from build123d import *

# Parameters (mm, degrees)
SKETCH1_W           = 25.4
SKETCH1_H           = 25.4
SKETCH1_W_2         = 19.05
SKETCH1_H_2         = 19.05
EXTRUDE_THIN1_DEPTH = 292.1
SKETCH4_R           = 2.4892
CUT_EXTRUDE1_DEPTH  = 26.4
CUT_EXTRUDE2_DEPTH  = 26.4
SKETCH3_R           = 3.175
CUT_EXTRUDE3_DEPTH  = 26.4


with BuildPart() as part:
    # Sketch1 → Extrude-Thin1 (new body, symmetric)
    with BuildSketch(Plane.XY):
        Rectangle(SKETCH1_W, SKETCH1_H)
        Rectangle(SKETCH1_W_2, SKETCH1_H_2, mode=Mode.SUBTRACT)
    extrude(amount=EXTRUDE_THIN1_DEPTH, both=True)

    # Sketch4 → Cut-Extrude1 (cut, through all)
    with BuildSketch(Plane.ZY.offset(12.7)):
        with Locations((266.7, 0)):
            Circle(SKETCH4_R)
        with Locations((139.7, 0)):
            Circle(SKETCH4_R)
        with Locations((234.949999999, 0)):
            Circle(SKETCH4_R)
    cut_extrude1 = extrude(amount=-CUT_EXTRUDE1_DEPTH, mode=Mode.SUBTRACT)

    # Mirror1: Cut-Extrude1 across plane
    add(cut_extrude1.mirror(Plane(origin=(0, 0, 0), x_dir=(1, 0, 0), z_dir=(0, 0, -1))), mode=Mode.SUBTRACT)

    # Sketch5 → Cut-Extrude2 (cut, through all)
    with BuildSketch(Plane.XZ.offset(12.7)):
        Polygon((12.7, -298.45), (12.7, -292.1), (-6.7e-08, -292.1), (-12.7, -292.1), (-12.7, -298.45), align=None)
        with BuildLine():
            ThreePointArc((-6.7e-08, -292.1), (-8.980256145, -288.380256097), (-12.7, -279.4))
            Line((-12.7, -279.4), (-12.7, -292.1))
            Line((-12.7, -292.1), (-6.7e-08, -292.1))
        make_face()
        with BuildLine():
            Line((12.7, -292.1), (12.7, -279.4))
            ThreePointArc((12.7, -279.4), (8.980256097, -288.380256145), (-6.7e-08, -292.1))
            Line((-6.7e-08, -292.1), (12.7, -292.1))
        make_face()
    extrude(amount=-CUT_EXTRUDE2_DEPTH, mode=Mode.SUBTRACT)

    # Sketch3 → Cut-Extrude3 (cut, through all)
    with BuildSketch(Plane(origin=(0, 12.7, 0), x_dir=(1, 0, 0), z_dir=(0, 1, 0))):
        with Locations((0, 279.4)):
            Circle(SKETCH3_R)
        with Locations((0, -279.4)):
            Circle(SKETCH3_R)
    extrude(amount=-CUT_EXTRUDE3_DEPTH, mode=Mode.SUBTRACT)


solid = part.part
For this review, take the finished solid that the model builds, in its own axes (mm). A direction names the side the tool comes from. Round coordinates to 2 decimals unless told otherwise and drop trailing zeros. Loops run counter-clockwise (first coordinate to the right, second up) from the corner with the lowest first, then second, coordinate; pieces in that order, holes last. Notation, with made-up numbers: (49, 79) - (106, 79) arc R27 cw to (106, 95) - close; hole circle Ø10 at (1, -13.5). An arc over 180 degrees is marked (long way). Use one line per item in the form item = value.
1) We need section A-A on z = 39.5. Write out the cut boundary in (x, y) (3 decimals), then the cut area to 3 significant figures.
Solutions:
outline = (-12.7, -12.7) - (12.7, -12.7) - (12.7, 12.7) - (-12.7, 12.7) - close; hole (-9.525, -9.525) - (9.525, -9.525) - (9.525, 9.525) - (-9.525, 9.525) - close
area = 282 mm2
2) Clearance check with a flat-ended pin moving along its axis: P1, Ø3, axis at y = 0, z = -234.95, coming from the -X side. State where the tip first meets the part, or that it passes through.
Solutions:
P1 = through
3) Tool access review of faces 5 (the face through (-12.7, 0, 10)), 6 (the face through (0, -9.525, 4)): name each direction out of +Z, -Z, +X, -X, +Y, -Y from which nothing blocks a thin tool from reaching the whole face with its end or side.
Solutions:
face_5 = +Z, -Z, -X, +Y, -Y
face_6 = +Z, -Z
4) Wall thickness on probe 1 along Z at (x, y) = (0, -10.15) (3 decimals); probe 2 along Y at (x, z) = (3.5, 99) (3 decimals): over which ranges is each line inside the solid? List them lowest first.
Solutions:
probe_1 = -292.1 to -282.575, -276.225 to 276.225, 282.575 to 292.1
probe_2 = -12.7 to -9.525, 9.525 to 12.7
5) Mouldability with a two-part tool opening along Y and no side actions: class faces 1 (the face through (9.525, 0, 6)), 2 (the face through (0, 9.525, 4)), 3 (the face through (11, 0, 292.1)), 4 (the face through (0, 12.7, 4)) as pulls with the +Y half, pulls with the -Y half, needs draft (parallel to the pull), parting line crosses it, or undercut.
Solutions:
face_1 = undercut
face_2 = undercut
face_3 = needs draft
face_4 = pulls with the +Y half
